Read the model definition and answer for the solid it produces. Units are mm, in the model's axes. Face numbers are marked on the shaded views. A direction names the side the tool comes from. Round coordinates to 2 decimals unless told otherwise and drop trailing zeros. Write each loop counter-clockwise with the first axis right and the second up, starting at its lowest first coordinate (ties: lowest second). Pieces come first, ordered by that corner, then holes. Notation, with made-up numbers: (60, 48.5) -> (87, 48.5) arc R24 ccw to (87, 80.5) -> close; hole circle Ø9 at (14.5, -33). An arc over 180 degrees is marked (long way). Return JSON: item names as keys, results as strings.
from build123d import *

# Parameters (mm, degrees)
F1_DEPTH  = 2
F2_R      = 2.5
F3_DEPTH  = 3
F4_R      = 1.4
F5_DEPTH  = 3
F6_R      = 1.4
F7_DEPTH  = 3
F8_R      = 1.4
F9_DEPTH  = 3.1
F10_R     = 1.4
F11_DEPTH = 3
F12_R     = 2.65
F12_W     = 54.34
F12_H     = 69.58
F13_DEPTH = 6.65
F14_R     = 1.75
F14_R_2   = 1.4
F15_DEPTH = 25
F16_W     = 13.04
F16_H     = 2.13
F16_W_2   = 10
F16_H_2   = 2.5
F17_DEPTH = 3
F18_SIZE  = 1
F20_DEPTH = 0.2


with BuildPart() as f1:
    # F0 (on Top) → F1 (new body)
    with BuildSketch(Plane.XY):
        with BuildLine():
            Line((55.84, 71.08), (-2.5, 71.08))
            ThreePointArc((-2.5, 71.08), (-8.156854, 68.736854), (-10.5, 63.08))
            Line((-10.5, 63.08), (-10.5, 5.5))
            ThreePointArc((-10.5, 5.5), (-8.156854, -0.156854), (-2.5, -2.5))
            Line((-2.5, -2.5), (55.84, -2.5))
            ThreePointArc((55.84, -2.5), (61.496854, -0.156854), (63.84, 5.5))
            Line((63.84, 5.5), (63.84, 63.08))
            ThreePointArc((63.84, 63.08), (61.496854, 68.736854), (55.84, 71.08))
        make_face()
    extrude(amount=F1_DEPTH)

    # F2 (on face) → F3 (join)
    with BuildSketch(Plane.XY.offset(2)):
        with Locations((17.78, 66.04)):
            Circle(F2_R)
        with Locations((45.72, 66.04)):
            Circle(F2_R)
        with Locations((2.54, 15.24)):
            Circle(F2_R)
        with Locations((50.8, 13.97)):
            Circle(F2_R)
    extrude(amount=F3_DEPTH)

    # F4 (on face) → F5 (join)
    with BuildSketch(Plane.XY.offset(5)):
        with Locations((17.78, 66.04)):
            Circle(F4_R)
    extrude(amount=F5_DEPTH)

    # F6 (on face) → F7 (join)
    with BuildSketch(Plane.XY.offset(5)):
        with Locations((45.72, 66.04)):
            Circle(F6_R)
    extrude(amount=F7_DEPTH)

    # F8 (on face) → F9 (join)
    with BuildSketch(Plane.XY.offset(5)):
        with Locations((2.54, 15.24)):
            Circle(F8_R)
    extrude(amount=F9_DEPTH)

    # F10 (on face) → F11 (join)
    with BuildSketch(Plane.XY.offset(5)):
        with Locations((50.8, 13.97)):
            Circle(F10_R)
    extrude(amount=F11_DEPTH)

    # F12 (on face) → F13 (join)
    with BuildSketch(Plane.XY.offset(2)):
        with BuildLine():
            ThreePointArc((-2.5, 71.08), (-8.156854, 68.736854), (-10.5, 63.08))
            Line((-10.5, 63.08), (-10.5, 5.5))
            ThreePointArc((-10.5, 5.5), (-8.156854, -0.156854), (-2.5, -2.5))
            Line((-2.5, -2.5), (55.84, -2.5))
            ThreePointArc((55.84, -2.5), (61.496854, -0.156854), (63.84, 5.5))
            Line((63.84, 5.5), (63.84, 63.08))
            ThreePointArc((63.84, 63.08), (61.496854, 68.736854), (55.84, 71.08))
            Line((55.84, 71.08), (-2.5, 71.08))
        make_face()
        with Locations((-5.5, 16.5)):
            Circle(F12_R, mode=Mode.SUBTRACT)
        with Locations((58.84, 16.5)):
            Circle(F12_R, mode=Mode.SUBTRACT)
        with Locations((-5.5, 52.08)):
            Circle(F12_R, mode=Mode.SUBTRACT)
        with Locations((26.67, 34.29)):
            Rectangle(F12_W, F12_H, mode=Mode.SUBTRACT)
        with Locations((58.84, 52.08)):
            Circle(F12_R, mode=Mode.SUBTRACT)
    extrude(amount=F13_DEPTH)

    # F14 (on face) → F15 (cut)
    with BuildSketch(Plane.XY.offset(8.65)):
        with Locations((-5.5, 9.5)):
            Circle(F14_R)
        with Locations((-4.5, 2.5)):
            Circle(F14_R_2)
        with Locations((-4.5, 66.08)):
            Circle(F14_R_2)
        with Locations((-5.5, 59.08)):
            Circle(F14_R)
        with Locations((57.84, 66.08)):
            Circle(F14_R_2)
        with Locations((58.84, 59.08)):
            Circle(F14_R)
        with Locations((58.84, 9.5)):
            Circle(F14_R)
        with Locations((57.84, 2.5)):
            Circle(F14_R_2)
    extrude(amount=-F15_DEPTH, mode=Mode.SUBTRACT)

    # F16 (on face) → F17 (cut)
    with BuildSketch(Plane.XZ.offset(2.5)):
        with Locations((15.02, 7.585)):
            Rectangle(F16_W, F16_H)
        with Locations((45.34, 7.4)):
            Rectangle(F16_W_2, F16_H_2)
    extrude(amount=-F17_DEPTH, mode=Mode.SUBTRACT)

    # F18
    f18_edges = [f1.edges().sort_by_distance(p)[0] for p in [
        (56.19, 16.5, 8.65),
        (56.19, 52.08, 8.65),
        (-8.15, 52.08, 8.65),
        (-8.15, 16.5, 8.65),
    ]]
    chamfer(f18_edges, length=F18_SIZE)

    # F19 (on face) → F20 (join)
    with BuildSketch(Plane(origin=(0, 0, 0), x_dir=(1, 0, 0), z_dir=(0, 0, -1))):
        with BuildLine():
            ThreePointArc((-2.5, 4.5), (-9.571068, 1.571068), (-12.5, -5.5))
            Line((-12.5, -5.5), (-12.5, -63.08))
            ThreePointArc((-12.5, -63.08), (-9.571068, -70.151068), (-2.5, -73.08))
            Line((-2.5, -73.08), (55.84, -73.08))
            ThreePointArc((55.84, -73.08), (62.911068, -70.151068), (65.84, -63.08))
            Line((65.84, -63.08), (65.84, -5.5))
            ThreePointArc((65.84, -5.5), (62.911068, 1.571068), (55.84, 4.5))
            Line((55.84, 4.5), (-2.5, 4.5))
        make_face()
        with BuildLine():
            Line((-10.5, -63.08), (-10.5, -5.5))
            ThreePointArc((-10.5, -5.5), (-8.156854, 0.156854), (-2.5, 2.5))
            Line((-2.5, 2.5), (55.84, 2.5))
            ThreePointArc((55.84, 2.5), (61.496854, 0.156854), (63.84, -5.5))
            Line((63.84, -5.5), (63.84, -63.08))
            ThreePointArc((63.84, -63.08), (61.496854, -68.736854), (55.84, -71.08))
            Line((55.84, -71.08), (-2.5, -71.08))
            ThreePointArc((-2.5, -71.08), (-8.156854, -68.736854), (-10.5, -63.08))
        make_face(mode=Mode.SUBTRACT)
    extrude(amount=-F20_DEPTH)


solid = f1.part
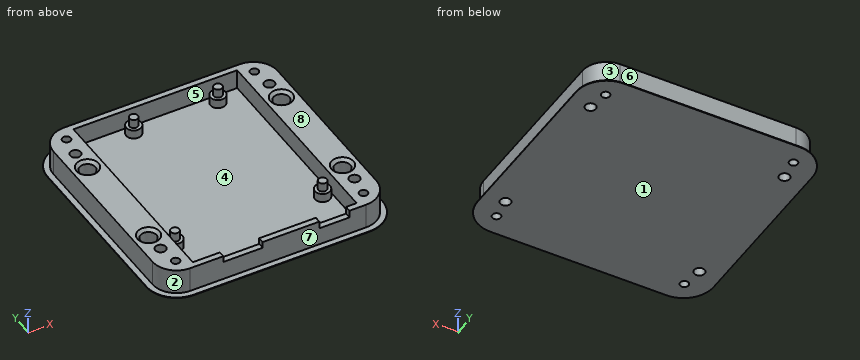
Item 1: A tool of negligible diameter and unlimited length cuts with its end or side. For the marked faces 5, 6, 7 and 8, from which of +Z, -Z, +X, -X, +Y, -Y can it reach the whole face along a straight path? Write none if from no direction.
Worked answers:
{"face 5": "+Z", "face 6": "+Z, +X, -X, +Y", "face 7": "+Z, +X, -X, -Y", "face 8": "+Z, +X, -X, +Y, -Y"}
Item 2: For a pull along X with two mould halves and no side action, classify the marked faces 1, 2, 3 and 4 as released by +X, released by -X, zero draft, split by the parting line, or undercut.
Worked answers:
{"face 1": "zero draft", "face 2": "released by -X", "face 3": "released by +X", "face 4": "undercut"}
Item 3: Flat-ended cylindrical pins translate along their axes: pin 1 (3 mm diameter, centred on x = 58.84, y = 16.5, fed in from +Z); pin 2 (4 mm diameter, centred on y = 43.5, z = 5.5, fed in from -X); pin 3 (1.5 mm diameter, centred on y = 27, z = 3, fed in from +X). Find the tip coordinate at first contact, or state that the pin passes through.
Worked answers:
{"pin 1": "stops at z = 2", "pin 2": "stops at x = -10.5", "pin 3": "stops at x = 63.84"}
Item 4: Section C-C (x = 9.5) is taken. Give the vertices of the cut face in (y, z).
Worked answers:
{"outline": "(-4.5, 0) -> (73.08, 0) -> (73.08, 0.2) -> (71.08, 0.2) -> (71.08, 8.65) -> (69.08, 8.65) -> (69.08, 2) -> (-0.5, 2) -> (-0.5, 6.52) -> (-2.5, 6.52) -> (-2.5, 0.2) -> (-4.5, 0.2) -> close"}
Item 5: Section A-A (z = 3.5) is taken. State how many separate pieces and enclosed holes the cut face has, then the cut area to 3 significant figures.
Worked answers:
{"separate pieces": "5", "enclosed holes": "13", "area": "1,560 mm2"}
Item 6: Section B-B (y = 31) is taken. Give the vertices of the cut face in (x, z), then the cut area to 3 significant figures.
Worked answers:
{"outline": "(-12.5, 0) -> (65.84, 0) -> (65.84, 0.2) -> (63.84, 0.2) -> (63.84, 8.65) -> (53.84, 8.65) -> (53.84, 2) -> (-0.5, 2) -> (-0.5, 8.65) -> (-10.5, 8.65) -> (-10.5, 0.2) -> (-12.5, 0.2) -> close", "area": "282 mm2"}
Item 7: Straight lines are drawn through the part: L1, parallel to X at y = 20.5, z = 4.25; L2, parallel to Y at x = 61, z = 3.25; L3, parallel to X at y = 11, z = 1.75. For each, find the intervals that lie inside material, in ascending order. Write a range as [from, to].
Worked answers:
{"L1": "x = [-10.5, -0.5], [53.84, 63.84]", "L2": "y = [-0.61, 14.96], [18.04, 50.54], [53.62, 69.19]", "L3": "x = [-10.5, -6.4], [-4.6, 57.94], [59.74, 63.84]"}
Item 8: Section D-D (x = 45.72) is taken. Give the vertices of the cut face in (y, z), then the cut area to 3 significant figures.
Worked answers:
{"outline": "(-4.5, 0) -> (73.08, 0) -> (73.08, 0.2) -> (71.08, 0.2) -> (71.08, 8.65) -> (69.08, 8.65) -> (69.08, 2) -> (68.54, 2) -> (68.54, 5) -> (67.44, 5) -> (67.44, 8) -> (64.64, 8) -> (64.64, 5) -> (63.54, 5) -> (63.54, 2) -> (-0.5, 2) -> (-0.5, 6.15) -> (-2.5, 6.15) -> (-2.5, 0.2) -> (-4.5, 0.2) -> close", "area": "193 mm2"}
